from build123d import *

# Parameters (mm, degrees)
SKETCH4_W           = 3.872983346
SKETCH4_H           = 1
BOSS_EXTRUDE1_DEPTH = 8
SKETCH5_R           = 2.5
BOSS_EXTRUDE2_DEPTH = 11


with BuildPart() as part:
    # Sketch2 → Revolve1 (revolve)
    with BuildSketch(Plane.XY, mode=Mode.PRIVATE) as revolve1_sk:
        Polygon((0, 0), (0, 50), (0, 53), (5, 53), (5, 50), (2.5, 50), (2.5, 5), (2, 5), (2, 0), align=None)
    revolve(revolve1_sk.sketch.rotate(Axis((0, 0, 0), (0, 1, 0)), 90), axis=Axis((0, 0, 0), (0, 1, 0)))

    # Sketch4 → Boss-Extrude1 (add)
    with BuildSketch(Plane.XZ):
        Rectangle(SKETCH4_W, SKETCH4_H)
    extrude(amount=BOSS_EXTRUDE1_DEPTH)

    # Sketch5 → Boss-Extrude2 (add)
    with BuildSketch(Plane(origin=(0, 53, 0), x_dir=(1, 0, 0), z_dir=(0, 1, 0))):
        with Locations(Location((0, 0, 0), (0, 0, 90))):
            Circle(SKETCH5_R)
    extrude(amount=BOSS_EXTRUDE2_DEPTH)


solid = part.part
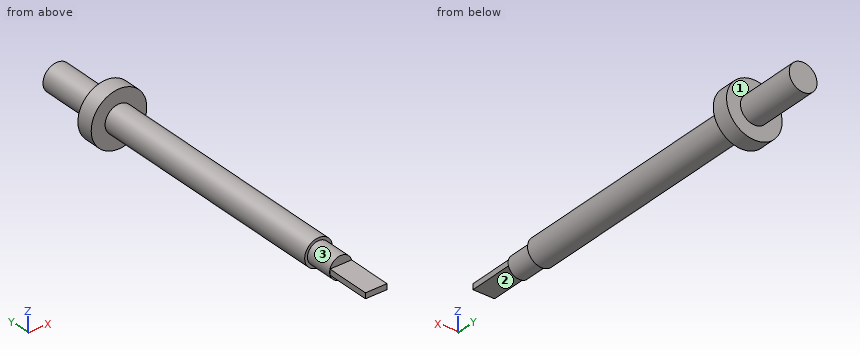
Can you work these out from the model? Positions are in its coordinate system, mm. Face numbers are marked on the shaded views. A direction names the side the tool comes from. Round coordinates to 2 decimals unless told otherwise and drop trailing zeros. Write each loop counter-clockwise with the first axis right and the second up, starting at its lowest first coordinate (ties: lowest second). Pieces come first, ordered by that corner, then holes. Notation, with made-up numbers: M -18,-5.5 L -9,-5.5 A35 cw -9,31.5 Z; hole C 66,5.25 d11. An arc over 180 degrees is marked long. Use a Markdown table: item, result.
Item 1: I want a section at A-A (x = 0). List the corners of the cut face in (y, z) for me.
Found:
| item | result |
|---|---|
| outline | M -8,-0.5 L 0,-0.5 L 0,-2 L 5,-2 L 5,-2.5 L 50,-2.5 L 50,-5 L 53,-5 L 53,-2.5 L 64,-2.5 L 64,2.5 L 53,2.5 L 53,5 L 50,5 L 50,2.5 L 5,2.5 L 5,2 L 0,2 L 0,0.5 L -8,0.5 Z |
Item 2: If I drill on line 1 along Y through (x, z) = (-2.75, -1.5); line 2 along Y through (x, z) = (0, -1.25); line 3 along Z through (x, y) = (-0.25, 51), over which ranges is the centre line in solid material (lowest first)? Write a range as [from, to].
Found:
| item | result |
|---|---|
| line 1 | y = [50, 53] |
| line 2 | y = [0, 64] |
| line 3 | z = [-4.99, 4.99] |
Item 3: I want a section at B-B (y = 2). List the corners of the cut face in (x, z) for me.
Found:
| item | result |
|---|---|
| outline | C 0,0 d4 |
Item 4: I want a section at C-C (z = 1.25). List the corners of the cut face in (x, y) for me, and give its area (3 significant figures).
Found:
| item | result |
|---|---|
| outline | M -4.84,50 L -2.17,50 L -2.17,5 L -1.56,5 L -1.56,0 L 1.56,0 L 1.56,5 L 2.17,5 L 2.17,50 L 4.84,50 L 4.84,53 L 2.17,53 L 2.17,64 L -2.17,64 L -2.17,53 L -4.84,53 Z |
| area | 287 mm2 |
Item 5: I want a section at D-D (y = 14). List the corners of the cut face in (x, z) for me, and give its area (3 significant figures).
Found:
| item | result |
|---|---|
| outline | C 0,0 d5 |
| area | 19.6 mm2 |
Item 6: For pin 1 Ø1.5 at (x, y) = (-2.5, 38.5) entering from -Z; pin 2 Ø6 at (y, z) = (46, -2) entering from +X; pin 3 Ø0.8 at (x, z) = (0, 1.5) entering from -Y, each with a flat end and sliding along its axis, tell me the tip position at first contact or that it passes through.
Found:
| item | result |
|---|---|
| pin 1 | stops at z = -1.79 |
| pin 2 | stops at x = 2.5 |
| pin 3 | stops at y = 0 |
Item 7: Which directions (+Z, -Z, +X, -X, +Y, -Y) give clear straight access to the entire face, cutting with the end or side of a thin tool? Please do the marked faces 1, 2 and 3.
Found:
| item | result |
|---|---|
| face 1 | +Y |
| face 2 | -Z, +X, -X, -Y |
| face 3 | -Y |
